Geometry check sheet. Reference: the model listing, model coordinates, mm. Face numbers are marked on the shaded views. Round coordinates to 2 decimals unless told otherwise and drop trailing zeros. Loops run counter-clockwise (first coordinate to the right, second up) from the corner with the lowest first, then second, coordinate; pieces in that order, holes last. Notation, with made-up numbers: (43.25, 79) -> (97.25, 79) arc R30 ccw to (97.25, 108) -> close; hole circle Ø6 at (1, 36). An arc over 180 degrees is marked (long way). Use one line per item in the form item = value.
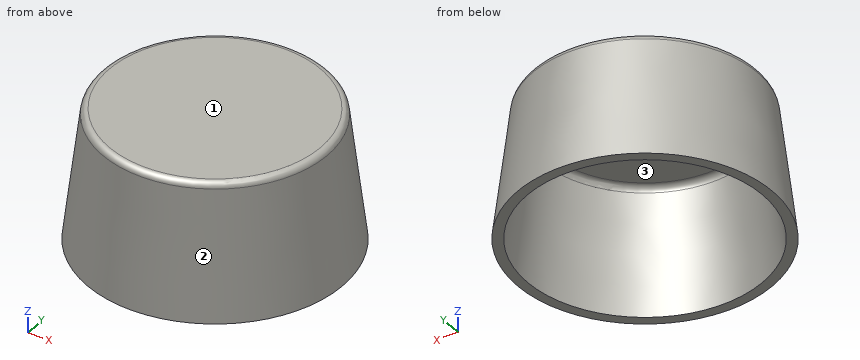
from build123d import *

# Parameters (mm, degrees)
F0_R     = 24.765
F1_DEPTH = 25.4
F1_TAPER = 7
F2_T     = -1.905
F3_R     = 1.27


with BuildPart() as f1:
    # F0 (on Top) → F1 (new body)
    with BuildSketch(Plane.XY):
        Circle(F0_R)
    extrude(amount=F1_DEPTH, taper=F1_TAPER)

    # F2
    f2_openings = [f1.faces().sort_by_distance(p)[0] for p in [
        (0, 0, 0),
    ]]
    offset(amount=F2_T, openings=f2_openings)

    # F3
    f3_edges = [f1.edges().sort_by_distance(p)[0] for p in [
        (-19.960871, 0, 23.495),
        (-21.646272, 0, 25.4),
    ]]
    fillet(f3_edges, radius=F3_R)


solid = f1.part
1. Gauge pin test, flat ends, axial feed: pin 1 (2 mm diameter, centred on y = 13, z = 6, fed in from +X); pin 2 (3 mm diameter, centred on y = -19, z = 5, fed in from +X); pin 3 (1.5 mm diameter, centred on x = -9.5, z = 3, fed in from +Y). Record the tip position at first contact, or that the pin passes through.
Return value:
pin_1 = 20.83
pin_2 = 16.67
pin_3 = 22.79
2. Section check D-D (z = 19.25). Record the boundary of the cut face in (x, y).
Return value:
outline = circle Ø44.8 at (0, 0); hole circle Ø40.96 at (0, 0)
3. Section check A-A (x = 0). Record the boundary of the cut face in (y, z) (3 decimals), then the cut area to 3 significant figures.
Return value:
outline = (-24.765, 0) -> (-22.846, 0) -> (-20.098, 22.38) arc R1.27 cw to (-18.837, 23.495) -> (18.837, 23.495) arc R1.27 cw to (20.098, 22.38) -> (22.846, 0) -> (24.765, 0) -> (21.783, 24.285) arc R1.27 ccw to (20.523, 25.4) -> (-20.523, 25.4) arc R1.27 ccw to (-21.783, 24.285) -> close
area = 173 mm2
4. Mould release check, pull along Y, two halves, no side actions. Record for the marked faces 1, 2 and 3: released by +Y, released by -Y, zero draft, split by the parting line, or undercut.
Return value:
face_1 = zero draft
face_2 = split by the parting line
face_3 = undercut
5. Section check C-C (z = 14.5). Record the boundary of the cut face in (x, y).
Return value:
outline = circle Ø45.97 at (0, 0); hole circle Ø42.13 at (0, 0)
6. Material ranges on line 1 along Z through (x, y) = (9.5, -5.5) (3 decimals); line 2 along X through (y, z) = (8, 23.25); line 3 along X through (y, z) = (7, 15), recorded low to high.
Return value:
line_1 = 23.495 to 25.4
line_2 = -20.4 to -17.88, 17.88 to 20.4
line_3 = -21.83 to -19.8, 19.8 to 21.83
